Source: three-view drawing plus pictorial views. Frame: mm from the lowest corner of the part. A direction names the side the tool comes from. Round coordinates to 2 decimals unless told otherwise and drop trailing zeros. Loops run counter-clockwise (first coordinate to the right, second up) from the corner with the lowest first, then second, coordinate; pieces in that order, holes last. Notation, with made-up numbers: M 62.5,50 L 103.5,50 A21 ccw 103.5,55 Z; hole C -24.5,47.25 d4. An arc over 180 degrees is marked long. Return JSON: item names as keys, results as strings. Group by question number.
1) Section D-D (z = 9.25). Output: boundary loops of the cut face in (x, y) (3 decimals).
2) Contact query for flat-ended pins moving along their axis: P1, Ø10, axis at x = 31.75, y = 6.35, coming from the +Z side; P2, Ø1.5, axis at y = 12.5, z = 6, coming from the -X side; P3, Ø5, axis at y = 20, z = 12.5, coming from the -X side. Output: stop coordinate, or through.
3) Access query for the marked faces 1 and 2. Directions: +Z, -Z, +X, -X, +Y, -Y. A direction counts if a zero-diameter tool reaches every point of the face in a straight line with its end or side. Return the directions, or none.
4) Mould query, pull axis X, two halves, no side actions, for the marked faces 3, 4, 5 and 6. Classes: +X half, -X half, draft (parallel to the pull), parting line (faces both ways), or undercut.
5) Section B-B (x = 31.75). Output: boundary loops of the cut face in (y, z) (3 decimals), plus the area to 3 significant figures.
6) Material intervals for line 1 (Z direction, x = 34.5, y = 54); line 2 (X direction, y = 60, z = 1.25); line 3 (Y direction, x = 6.35, z = 4.25) (3 decimals), sorted ascending. Write a range as from..to.
7) Section A-A (x = 57.15). Output: boundary loops of the cut face in (y, z) (3 decimals), plus the area to 3 significant figures.
8) Section C-C (y = 38.5). Output: boundary loops of the cut face in (x, z), plus the area to 3 significant figures.
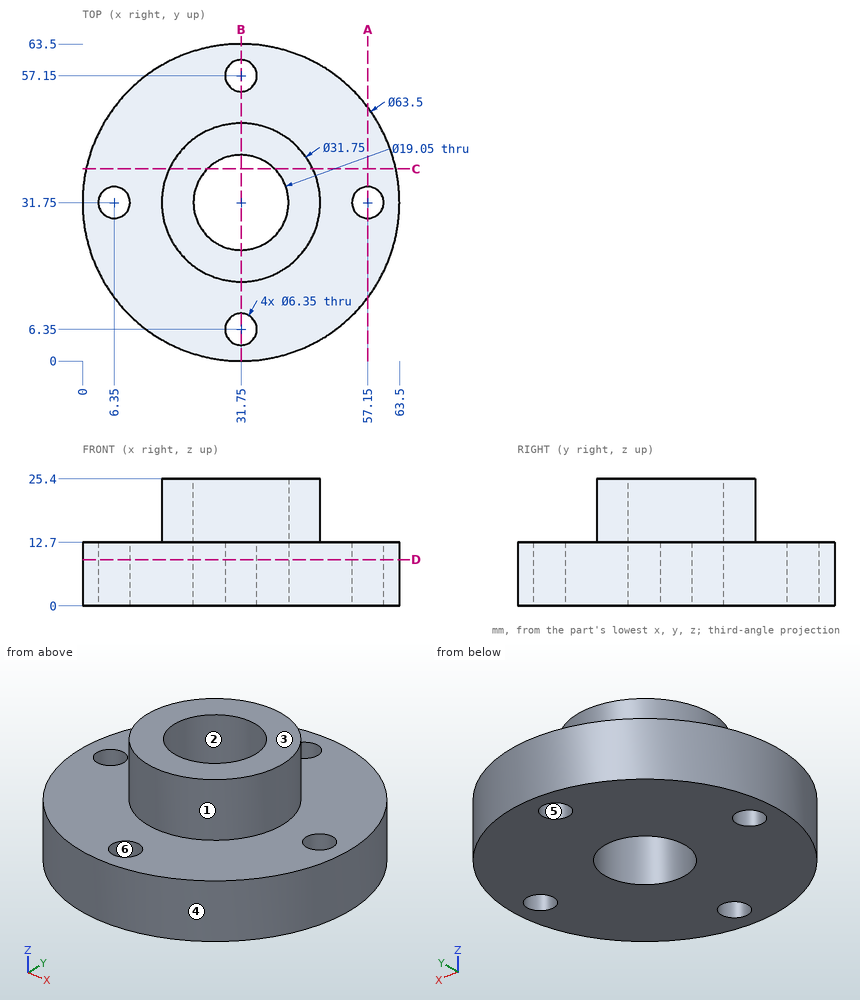
Returned:
{
 "1": {"outline": "C 31.75,31.75 d63.5; hole C 6.35,31.75 d6.35; hole C 31.75,31.75 d19.05; hole C 31.75,6.35 d6.35; hole C 31.75,57.15 d6.35; hole C 57.15,31.75 d6.35"},
 "2": {"P1": "stops at z = 12.7", "P2": "stops at x = 5.95", "P3": "stops at x = 1.38"},
 "3": {"face 1": "+Z", "face 2": "+Z, -Z"},
 "4": {"face 3": "draft", "face 4": "parting line", "face 5": "undercut", "face 6": "undercut"},
 "5": {"outline": "M 0,0 L 3.175,0 L 3.175,12.7 L 0,12.7 Z; M 9.525,0 L 22.225,0 L 22.225,25.4 L 15.875,25.4 L 15.875,12.7 L 9.525,12.7 Z; M 41.275,0 L 53.975,0 L 53.975,12.7 L 47.625,12.7 L 47.625,25.4 L 41.275,25.4 Z; M 60.325,0 L 63.5,0 L 63.5,12.7 L 60.325,12.7 Z", "area": "565 mm^2"},
 "6": {"line 1": "z = 0..12.7", "line 2": "x = 17.26..30.35, 33.15..46.24", "line 3": "y = 12.7..28.575, 34.925..50.8"},
 "7": {"outline": "M 12.7,0 L 28.575,0 L 28.575,12.7 L 12.7,12.7 Z; M 34.925,0 L 50.8,0 L 50.8,12.7 L 34.925,12.7 Z", "area": "403 mm^2"},
 "8": {"outline": "M 0.73,0 L 25.03,0 L 25.03,25.4 L 17.38,25.4 L 17.38,12.7 L 0.73,12.7 Z; M 38.47,0 L 62.77,0 L 62.77,12.7 L 46.12,12.7 L 46.12,25.4 L 38.47,25.4 Z", "area": "812 mm^2"}
}
